Answer from the drawing. Dimensions are ordinates in mm from the lowest x, y and z of the part. A direction names the side the tool comes from. Round coordinates to 2 decimals unless told otherwise and drop trailing zeros. Order: outer loops, then holes, each group sorted by start corner. A loop starts at its lowest first (then second) coordinate and runs counter-clockwise, first axis right, second up. Notation, with made-up numbers: (-24, -20.75) -> (3, -20.75) arc R27 cw to (3, 16.25) -> close; hole circle Ø4 at (19, 37.25). An arc over 180 degrees is marked (long way). Use a Markdown table: item, result. Add a question column.
Item 1: A cutting plane is placed at D-D, the plane y = 2.25. Determine the outline of the cut face in (x, z), plus the area to 3 significant figures.
Item 2: A cutting plane is placed at B-B, the plane x = 18.5. Determine the outline of the cut face in (y, z).
Item 3: A cutting plane is placed at A-A, the plane x = 14. Determine the outline of the cut face in (y, z), plus the area to 3 significant figures.
Item 4: A cutting plane is placed at C-C, the plane z = 5.75. Determine the outline of the cut face in (x, y), plus the area to 3 significant figures.
Item 5: For a pull along X with two mould halves and no side action, classify the marked faces 1, 2 and 3 as +X half, -X half, draft (parallel to the pull), parting line (faces both ways), or undercut.
Item 6: Find the intervals of material crossed by L1, parallel to Z at x = 9.75, y = 1.75; L2, parallel to X at y = 8, z = 21.25; L3, parallel to Z at x = 14.5, y = 3, in increasing order. Write a range as [from, to].
Item 7: A tool of negligible diameter and unlimited length cuts with its end or side. For the marked faces 4, 5 and 6, from which of +Z, -Z, +X, -X, +Y, -Y can it reach the whole face along a straight path? Write none if from no direction.
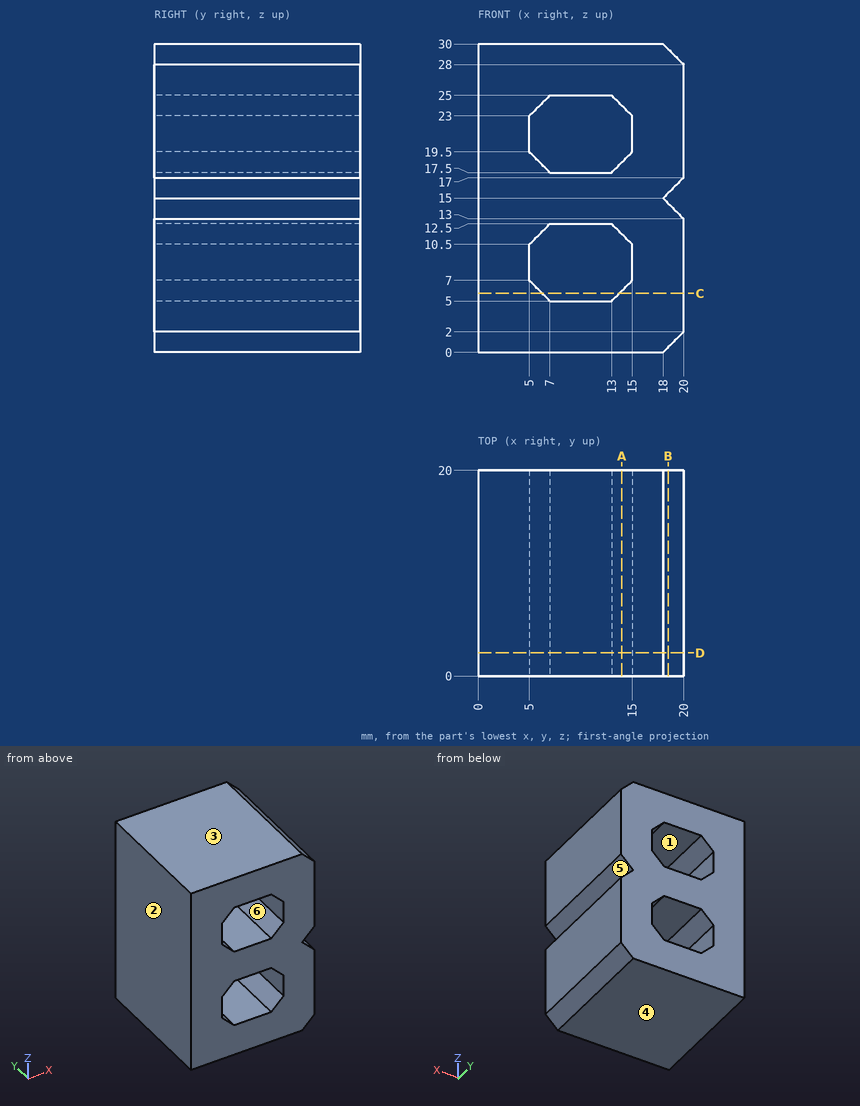
Reported:
| question | item | result |
|---|---|---|
| 1 | outline | (0, 0) -> (18, 0) -> (20, 2) -> (20, 13) -> (18, 15) -> (20, 17) -> (20, 28) -> (18, 30) -> (0, 30) -> close; hole (5, 7) -> (7, 5) -> (13, 5) -> (15, 7) -> (15, 10.5) -> (13, 12.5) -> (7, 12.5) -> (5, 10.5) -> close; hole (5, 19.5) -> (7, 17.5) -> (13, 17.5) -> (15, 19.5) -> (15, 23) -> (13, 25) -> (7, 25) -> (5, 23) -> close |
| 1 | area | 458 mm² |
| 2 | outline | (0, 0.5) -> (20, 0.5) -> (20, 14.5) -> (0, 14.5) -> close; (0, 15.5) -> (20, 15.5) -> (20, 29.5) -> (0, 29.5) -> close |
| 3 | outline | (0, 0) -> (20, 0) -> (20, 6) -> (0, 6) -> close; (0, 11.5) -> (20, 11.5) -> (20, 18.5) -> (0, 18.5) -> close; (0, 24) -> (20, 24) -> (20, 30) -> (0, 30) -> close |
| 3 | area | 380 mm² |
| 4 | outline | (0, 0) -> (6.25, 0) -> (6.25, 20) -> (0, 20) -> close; (13.75, 0) -> (20, 0) -> (20, 20) -> (13.75, 20) -> close |
| 4 | area | 250 mm² |
| 5 | face 1 | undercut |
| 5 | face 2 | -X half |
| 5 | face 3 | draft |
| 6 | L1 | [0, 5], [12.5, 17.5], [25, 30] |
| 6 | L2 | [0, 5], [15, 20] |
| 6 | L3 | [0, 6.5], [11, 19], [23.5, 30] |
| 7 | face 4 | -Z, +X, -X, +Y, -Y |
| 7 | face 5 | +X, +Y, -Y |
| 7 | face 6 | +Y, -Y |
